Work out the finished part from the listing and answer in its coordinate system (mm). Face numbers are marked on the shaded views. Round coordinates to 2 decimals unless told otherwise and drop trailing zeros. Loops run counter-clockwise (first coordinate to the right, second up) from the corner with the lowest first, then second, coordinate; pieces in that order, holes last. Notation, with made-up numbers: (85.5, 9) -> (133.5, 9) arc R24 ccw to (133.5, 46) -> close; hole circle Ø10 at (-12, 71). An arc over 180 degrees is marked (long way). Use CSV: the item, a comma, the result in double quotes. Start each with the question number.
from build123d import *

# Parameters (mm, degrees)
BOSS_EXTRUDE1_DEPTH = 10
SKETCH8_R           = 2
CUT_EXTRUDE10_DEPTH = 21
SKETCH10_R          = 3
CUT_EXTRUDE11_DEPTH = 3
SKETCH11_R          = 2.25
CUT_EXTRUDE12_DEPTH = 12
SKETCH20_R          = 57.5
SKETCH20_R_2        = 2.25
SKETCH20_R_3        = 3
CUT_EXTRUDE20_DEPTH = 1
CUT_EXTRUDE23_DEPTH = 153
SKETCH27_R          = 10
CUT_EXTRUDE24_DEPTH = 153
FILLET8_R           = 20
FILLET9_R           = 5


with BuildPart() as part:
    # Sketch1 → Boss-Extrude1 (new body)
    with BuildSketch(Plane(origin=(0, 0, 0), x_dir=(1, 0, 0), z_dir=(0, 1, 0))):
        Polygon((92.37604307, 0), (46.188021535, 80), (-46.188021535, 80), (-92.37604307, 0), (-46.188021535, -80), (46.188021535, -80), align=None)
    extrude(amount=BOSS_EXTRUDE1_DEPTH)

    # Sketch8 → Cut-Extrude10 (cut)
    with BuildSketch(Plane(origin=(0, 10, 0), x_dir=(1, 0, 0), z_dir=(0, 1, 0))):
        with Locations((-42.5, 15)):
            Circle(SKETCH8_R)
        with Locations((-42.5, -15)):
            Circle(SKETCH8_R)
        with Locations((42.5, 15)):
            Circle(SKETCH8_R)
        with Locations((42.5, -15)):
            Circle(SKETCH8_R)
    extrude(amount=-CUT_EXTRUDE10_DEPTH, mode=Mode.SUBTRACT)

    # Sketch10 → Cut-Extrude11 (cut)
    with BuildSketch(Plane(origin=(0, 10, 0), x_dir=(1, 0, 0), z_dir=(0, 1, 0))):
        with Locations((-42.5, 15)):
            Circle(SKETCH10_R)
        with Locations((-42.5, -15)):
            Circle(SKETCH10_R)
        with Locations((42.5, 15)):
            Circle(SKETCH10_R)
        with Locations((42.5, -15)):
            Circle(SKETCH10_R)
    extrude(amount=-CUT_EXTRUDE11_DEPTH, mode=Mode.SUBTRACT)

    # Sketch11 → Cut-Extrude12 (cut)
    with BuildSketch(Plane(origin=(0, 10, 0), x_dir=(1, 0, 0), z_dir=(0, 1, 0))):
        with Locations((-40, 30)):
            Circle(SKETCH11_R)
        with Locations((-40, -30)):
            Circle(SKETCH11_R)
        with Locations((40, -30)):
            Circle(SKETCH11_R)
        with Locations((40, 30)):
            Circle(SKETCH11_R)
    extrude(amount=-CUT_EXTRUDE12_DEPTH, mode=Mode.SUBTRACT)

    # Sketch20 → Cut-Extrude20 (cut)
    with BuildSketch(Plane(origin=(0, 10, 0), x_dir=(1, 0, 0), z_dir=(0, 1, 0))):
        Circle(SKETCH20_R)
        with Locations((40, 30)):
            Circle(SKETCH20_R_2, mode=Mode.SUBTRACT)
        with Locations((-40, -30)):
            Circle(SKETCH20_R_2, mode=Mode.SUBTRACT)
        with Locations((42.5, -15)):
            Circle(SKETCH20_R_3, mode=Mode.SUBTRACT)
        with Locations((-42.5, -15)):
            Circle(SKETCH20_R_3, mode=Mode.SUBTRACT)
        with Locations((-42.5, 15)):
            Circle(SKETCH20_R_3, mode=Mode.SUBTRACT)
        with Locations((42.5, 15)):
            Circle(SKETCH20_R_3, mode=Mode.SUBTRACT)
        with Locations((-40, 30)):
            Circle(SKETCH20_R_2, mode=Mode.SUBTRACT)
        with Locations((40, -30)):
            Circle(SKETCH20_R_2, mode=Mode.SUBTRACT)
    extrude(amount=-CUT_EXTRUDE20_DEPTH, mode=Mode.SUBTRACT)

    # Sketch20_7 → Cut-Extrude23 (cut)
    with BuildSketch(Plane(origin=(0, 10, 0), x_dir=(1, 0, 0), z_dir=(0, 1, 0))):
        with BuildLine():
            Line((-51.265241636, 51.265241636), (-40.658639918, 40.658639918))
            ThreePointArc((-40.658639918, 40.658639918), (0, 57.5), (40.658639918, 40.658639918))
            Line((40.658639918, 40.658639918), (51.265241636, 51.265241636))
            ThreePointArc((51.265241636, 51.265241636), (0, 72.5), (-51.265241636, 51.265241636))
        make_face()
        with BuildLine():
            ThreePointArc((40.658639918, -40.658639918), (0, -57.5), (-40.658639918, -40.658639918))
            Line((-40.658639918, -40.658639918), (-51.265241636, -51.265241636))
            ThreePointArc((-51.265241636, -51.265241636), (0, -72.5), (51.265241636, -51.265241636))
            Line((51.265241636, -51.265241636), (40.658639918, -40.658639918))
        make_face()
    extrude(amount=-CUT_EXTRUDE23_DEPTH, mode=Mode.SUBTRACT)

    # Sketch27 → Cut-Extrude24 (cut)
    with BuildSketch(Plane(origin=(0, 9, 0), x_dir=(1, 0, 0), z_dir=(0, 1, 0))):
        with Locations((0, -42)):
            Circle(SKETCH27_R)
        with Locations((0, 42)):
            Circle(SKETCH27_R)
    extrude(amount=-CUT_EXTRUDE24_DEPTH, mode=Mode.SUBTRACT)

    # Fillet8
    fillet8_edges = [part.edges().sort_by_distance(p)[0] for p in [
        (-92.37604307, 5, 0),
        (92.37604307, 5, 0),
    ]]
    fillet(fillet8_edges, radius=FILLET8_R)

    # Fillet9
    fillet9_edges = [part.edges().sort_by_distance(p)[0] for p in [
        (46.188021535, 5, 80),
        (-46.188021535, 5, 80),
        (-46.188021535, 5, -80),
        (46.188021535, 5, -80),
    ]]
    fillet(fillet9_edges, radius=FILLET9_R)


solid = part.part
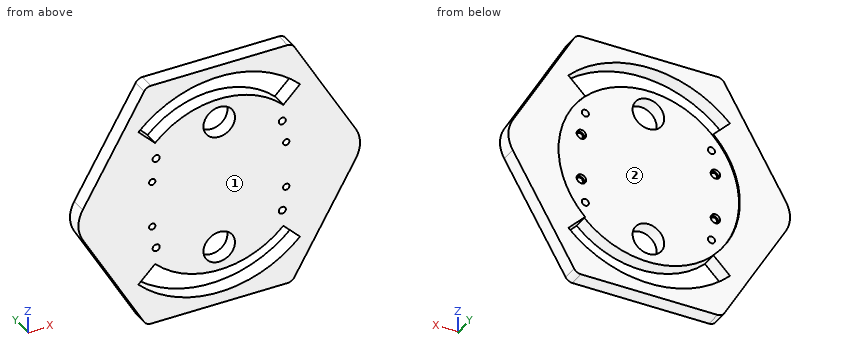
Q1. Section D-D, the plane x = 24 is taken. Write down the section's boundary in (y, z), and give its area (3 significant figures).
Q2. Section C-C, the plane z = 15 is taken. Write down the section's boundary in (x, y).
Q3. For a pull along Z with two mould halves and no side action, classify the marked faces 1 and 2 as pulls with the +Z half, pulls with the -Z half, needs draft (parallel to the pull), parting line crosses it, or undercut.
Q4. Section A-A, the plane y = 1.5 is taken. Give the number of separate pieces and of enclosed holes in the cut face, and give its area (3 significant figures).
Q5. Each of these flat-tipped pins is pushed along its axis until it touches: pin 1 (2 mm diameter, centred on y = 5.5, z = -23, fed in from -X); pin 2 (2 mm diameter, centred on y = 7, z = 48.5, fed in from +X); pin 3 (6.5 mm diameter, centred on x = -43.5, z = -14.5, fed in from +Y). Where does it stop, or does it pass through?
Q6. Section B-B, the plane x = 0 is taken. Write down the section's boundary in (y, z).
Q7. Straight lines are drawn through the part: line 1 (Z direction, x = -42.5, y = 7.75); line 2 (Z direction, x = 23, y = 8.75) (3 decimals); line 3 (Z direction, x = 0, y = 6.5). For each, find the intervals that lie inside material, in ascending order. Write a range as from..to.
Report:
1,outline,"(0, -80) -> (10, -80) -> (10, -68.41) -> (0, -68.41) -> close; (0, -52.25) -> (9, -52.25) -> (9, 52.25) -> (0, 52.25) -> close; (0, 68.41) -> (10, 68.41) -> (10, 80) -> (0, 80) -> close"
1,area,"1,170 mm²"
2,outline,"(-83.72, 0) -> (-44.5, 0) -> (-44.5, 7) -> (-45.5, 7) -> (-45.5, 9) -> (-55.51, 9) -> (-55.51, 10) -> (-83.72, 10) -> close; (-40.5, 0) -> (40.5, 0) -> (40.5, 7) -> (39.5, 7) -> (39.5, 9) -> (-39.5, 9) -> (-39.5, 7) -> (-40.5, 7) -> close; (44.5, 0) -> (83.72, 0) -> (83.72, 10) -> (55.51, 10) -> (55.51, 9) -> (45.5, 9) -> (45.5, 7) -> (44.5, 7) -> close"
3,face 1,"needs draft"
3,face 2,"undercut"
4,separate pieces,"1"
4,enclosed holes,"12"
4,area,"18,300 mm²"
5,pin 1,"stops at x = -79.67"
5,pin 2,"stops at x = 64.95"
5,pin 3,"stops at y = 9"
6,outline,"(0, -80) -> (10, -80) -> (10, -72.5) -> (0, -72.5) -> close; (0, -57.5) -> (9, -57.5) -> (9, -52) -> (0, -52) -> close; (0, -32) -> (9, -32) -> (9, 32) -> (0, 32) -> close; (0, 52) -> (9, 52) -> (9, 57.5) -> (0, 57.5) -> close; (0, 72.5) -> (10, 72.5) -> (10, 80) -> (0, 80) -> close"
7,line 1,"z = -80..-58.74, -42.5..-18, -12..12, 18..42.5, 58.74..80"
7,line 2,"z = -80..-68.755, -52.7..52.7, 68.755..80"
7,line 3,"z = -80..-72.5, -57.5..-52, -32..32, 52..57.5, 72.5..80"
